from build123d import *

# Parameters (mm, degrees)
SKETCH1_R           = 4.5
BOSS_EXTRUDE2_DEPTH = 5
SKETCH2_W           = 5
SKETCH2_H           = 2.5
BOSS_EXTRUDE3_DEPTH = 10
SKETCH3_W           = 10
SKETCH3_H           = 2.5
BOSS_EXTRUDE4_DEPTH = 5
SKETCH4_W           = 10
SKETCH4_H           = 2.5
BOSS_EXTRUDE5_DEPTH = 5
SKETCH5_R           = 1.65
CUT_EXTRUDE1_DEPTH  = 5
CHAMFER1_SIZE       = 5.773502692
CHAMFER1_SIZE_2     = 10
FILLET1_R           = 2
FILLET2_R           = 5
FILLET3_R           = 2
FILLET4_R           = 2
FILLET5_R           = 10
FILLET6_R           = 3
SKETCH6_R           = 1.65
SKETCH6_W           = 36.073404507
SKETCH6_H           = 7.954648173
CUT_EXTRUDE2_DEPTH  = 5
FILLET10_R          = 2


with BuildPart() as part:
    # Sketch1 → Boss-Extrude2 (new body)
    with BuildSketch(Plane.XY):
        with BuildLine():
            Line((-7.5, 20), (-5.870329309, 16.740658618))
            ThreePointArc((-5.870329309, 16.740658618), (0, 21.5), (5.870329309, 16.740658618))
            Line((5.870329309, 16.740658618), (7.5, 20))
            Line((7.5, 20), (12.5, 20))
            Line((12.5, 20), (12.5, 15))
            Line((12.5, 15), (5, 0))
            Line((5, 0), (12.5, -15))
            Line((12.5, -15), (12.5, -20))
            Line((12.5, -20), (7.5, -20))
            Line((7.5, -20), (0, -5))
            Line((0, -5), (-7.5, -20))
            Line((-7.5, -20), (-12.5, -20))
            Line((-12.5, -20), (-12.5, -15))
            Line((-12.5, -15), (-5, 0))
            Line((-5, 0), (-12.5, 15))
            Line((-12.5, 15), (-12.5, 20))
            Line((-12.5, 20), (-7.5, 20))
        make_face()
        with Locations((0, 15.5)):
            Circle(SKETCH1_R, mode=Mode.SUBTRACT)
    extrude(amount=BOSS_EXTRUDE2_DEPTH)

    # Sketch2 → Boss-Extrude3 (add)
    with BuildSketch(Plane.XY.offset(5)):
        with Locations((-10, -18.75)):
            Rectangle(SKETCH2_W, SKETCH2_H)
        with Locations((10, -18.75)):
            Rectangle(SKETCH2_W, SKETCH2_H)
    extrude(amount=BOSS_EXTRUDE3_DEPTH)

    # Sketch3 → Boss-Extrude4 (add)
    with BuildSketch(Plane(origin=(12.5, 0, 0), x_dir=(0, 0, -1), z_dir=(1, 0, 0))):
        with Locations((-5, -18.75)):
            Rectangle(SKETCH3_W, SKETCH3_H)
    extrude(amount=BOSS_EXTRUDE4_DEPTH)

    # Sketch4 → Boss-Extrude5 (add)
    with BuildSketch(Plane.ZY.offset(12.5)):
        with Locations((5, -18.75)):
            Rectangle(SKETCH4_W, SKETCH4_H)
    extrude(amount=BOSS_EXTRUDE5_DEPTH)

    # Sketch5 → Cut-Extrude1 (cut)
    with BuildSketch(Plane(origin=(0, -17.5, 0), x_dir=(1, 0, 0), z_dir=(0, 1, 0))):
        with Locations(Location((-15, -3, 0), (0, 0, 270))):
            Circle(SKETCH5_R)
        with Locations(Location((-10, -12, 0), (0, 0, 270))):
            Circle(SKETCH5_R)
        with Locations(Location((10, -12, 0), (0, 0, 270))):
            Circle(SKETCH5_R)
        with Locations(Location((15, -3, 0), (0, 0, 270))):
            Circle(SKETCH5_R)
    extrude(amount=-CUT_EXTRUDE1_DEPTH, mode=Mode.SUBTRACT)

    # Chamfer1
    # the kernel refuses this chamfer: 10, 5.773502692 mm, written as the material it takes off along each edge
    with BuildSketch(Plane(origin=(17.5, -45.870857546, 10), x_dir=(0.05789386240267053, 0, -0.9983227437537926), z_dir=(0, 1, 0))) as chamfer1_piece_1_section:
        Polygon((CHAMFER1_SIZE * 0.998322743736, CHAMFER1_SIZE * 0.0578938624016), (-CHAMFER1_SIZE_2 * 0.0578938624027, CHAMFER1_SIZE_2 * 0.998322743754), (0, 0), align=None)
    chamfer1_piece_1 = extrude(amount=54.241715093, mode=Mode.PRIVATE)
    chamfer1_piece_1 = split(chamfer1_piece_1, bisect_by=Plane(origin=(12.5, -18.75, 7.760588383), z_dir=(1, 0, 0)), keep=Keep.TOP, mode=Mode.PRIVATE)
    add(chamfer1_piece_1, mode=Mode.SUBTRACT)
    with BuildSketch(Plane(origin=(-17.5, -45.870857546, 10), x_dir=(-0.05789386240267053, 0, -0.9983227437537926), z_dir=(0, 1, 0))) as chamfer1_piece_2_section:
        Polygon((CHAMFER1_SIZE * 0.998322743736, -CHAMFER1_SIZE * 0.0578938624016), (-CHAMFER1_SIZE_2 * 0.0578938624027, -CHAMFER1_SIZE_2 * 0.998322743754), (0, 0), align=None)
    chamfer1_piece_2 = extrude(amount=54.241715093, mode=Mode.PRIVATE)
    chamfer1_piece_2 = split(chamfer1_piece_2, bisect_by=Plane(origin=(-12.5, -18.75, 7.760588383), z_dir=(-1, 0, 0)), keep=Keep.TOP, mode=Mode.PRIVATE)
    add(chamfer1_piece_2, mode=Mode.SUBTRACT)

    # Fillet1
    fillet1_edges = [part.edges().sort_by_distance(p)[0] for p in [
        (12.5, -18.75, 15),
        (7.5, -18.75, 15),
        (-7.5, -18.75, 15),
        (-12.5, -18.75, 15),
    ]]
    fillet(fillet1_edges, radius=FILLET1_R)

    # Fillet2
    fillet2_edges = [part.edges().sort_by_distance(p)[0] for p in [
        (12.5, -18.75, 7.113248654),
        (-12.5, -18.75, 7.113248654),
    ]]
    fillet(fillet2_edges, radius=FILLET2_R)

    # Fillet3
    fillet3_edges = [part.edges().sort_by_distance(p)[0] for p in [
        (17.5, -18.75, 4.226497308),
        (-17.5, -18.75, 4.226497308),
    ]]
    fillet(fillet3_edges, radius=FILLET3_R)

    # Fillet4
    # the kernel refuses this fillet: 2 mm, written as the material it adds along each edge
    with BuildSketch(Plane(origin=(-5.870329309, 16.740658618, 0), x_dir=(-0.4472135954999439, 0.894427190999923, 0), z_dir=(0, 0, 1))) as fillet4_piece_1:
        with BuildLine():
            CenterArc((3.795112325, -1.99428722), FILLET4_R, 94.331614503, 105.404093699)
            Line((1.912591774, -2.669651103), (1.874941363, -2.683158381))
            ThreePointArc((1.874941363, -2.683158381), (1.109985705, -1.224719073), (-0.024899799, -0.031304952))
            Line((-0.024899799, -0.031304952), (0, 0.04))
            ThreePointArc((0, 0.04), (1.822027223, 0.04), (3.641033289, 0.039885744))
            Line((3.641033289, 0.039885744), (3.644054446, 0))
        make_face()
    extrude(amount=5)
    with BuildSketch(Plane(origin=(5.870329309, 16.740658618, 0), x_dir=(-0.46663943526551355, 0.8844476454008358, 0), z_dir=(0, 0, 1))) as fillet4_piece_2:
        with BuildLine():
            CenterArc((3.831402307, -1.923646391), FILLET4_R, 105.88286544, 105.404093699)
            Line((2.1222482, -2.962295628), (2.088065118, -2.983068612))
            ThreePointArc((2.088065118, -2.983068612), (1.02860762, -1.504443275), (-0.03251648, -0.023295461))
            Line((-0.03251648, -0.023295461), (0.010946864, 0.038472928))
            ThreePointArc((0.010946864, 0.038472928), (1.64202956, -0.189060828), (3.273112257, 0.038472928))
            Line((3.273112257, 0.038472928), (3.284059121, 0))
        make_face()
    extrude(amount=5)
    with BuildSketch(Plane(origin=(0, -5, 0), x_dir=(-0.4472135954999584, -0.8944271909999157, 0), z_dir=(0, 0, 1))) as fillet4_piece_3:
        with BuildLine():
            CenterArc((FILLET4_R * 2, FILLET4_R), FILLET4_R, 143.130102354, 126.869897646)
            Line((FILLET4_R * 1.2, FILLET4_R * 1.6), (FILLET4_R * 1.184, FILLET4_R * 1.612))
            Line((FILLET4_R * 1.184, FILLET4_R * 1.612), (-FILLET4_R * 0.016, FILLET4_R * 0.012))
            Line((-FILLET4_R * 0.016, FILLET4_R * 0.012), (0, -FILLET4_R * 0.02))
            Line((0, -FILLET4_R * 0.02), (FILLET4_R * 2, -FILLET4_R * 0.02))
            Line((FILLET4_R * 2, -FILLET4_R * 0.02), (FILLET4_R * 2, 0))
        make_face()
    extrude(amount=5)

    # Fillet5
    fillet5_edges = [part.edges().sort_by_distance(p)[0] for p in [
        (5, 0, 2.5),
        (-5, 0, 2.5),
    ]]
    fillet(fillet5_edges, radius=FILLET5_R)

    # Fillet6
    fillet6_edges = [part.edges().sort_by_distance(p)[0] for p in [
        (7.5, 20, 2.5),
        (12.5, 20, 2.5),
        (12.5, 15, 2.5),
        (-12.5, 15, 2.5),
        (-12.5, 20, 2.5),
        (-7.5, 20, 2.5),
    ]]
    fillet(fillet6_edges, radius=FILLET6_R)

    # Sketch6 → Cut-Extrude2 (cut)
    with BuildSketch(Plane(origin=(0, -17.5, 0), x_dir=(1, 0, 0), z_dir=(0, 1, 0))):
        with Locations(Location((-10, -7.5, 0), (0, 0, 270))):
            Circle(SKETCH6_R)
        with Locations(Location((10, -7.5, 0), (0, 0, 270))):
            Circle(SKETCH6_R)
        with Locations((1.341190681, -13.977324087)):
            Rectangle(SKETCH6_W, SKETCH6_H)
    extrude(amount=-CUT_EXTRUDE2_DEPTH, mode=Mode.SUBTRACT)

    # Fillet10
    fillet10_edges = [part.edges().sort_by_distance(p)[0] for p in [
        (12.5, -18.75, 10),
        (-12.5, -18.75, 10),
        (7.5, -18.75, 10),
        (-7.5, -18.75, 10),
    ]]
    fillet(fillet10_edges, radius=FILLET10_R)


solid = part.part
Model file for the job. Use its own axes, mm. A direction names the side the tool comes from. Coordinates: 2 decimals unless noted, no trailing zeros. Write each loop counter-clockwise with the first axis right and the second up, starting at its lowest first coordinate (ties: lowest second). Pieces come first, ordered by that corner, then holes. Notation, with made-up numbers: (14.25, 10.5) -> (26.25, 10.5) arc R25 cw to (26.25, 28.5) -> close; hole circle Ø7 at (-5.75, 55). An arc over 180 degrees is marked (long way). One line per item, written item: value. Start each with the question number.
1) Slice it at B-B on y = -6. Write the cut outline in (x, z), then the cut area to 3 significant figures.
2) Slice it at C-C on x = -10. Write the cut outline in (y, z), then the cut area to 3 significant figures.
3) Slice it at D-D on z = 2.25. Count the separate pieces of the cut face and the enclosed holes in it, then the cut area to 3 significant figures.
4) Pull direction Z, two halves, no side cores. Call faces 1 (the face through (-11, -18.73, 6.19)), 2 (the face through (13, -17.5, 5)), 3 (the face through (10, -19, 10)): +Z half, -Z half, draft (parallel to the pull), parting line (faces both ways), or undercut.
5) Probe probe 1 along X at (y, z) = (-18.55, 7.5); probe 2 along Z at (x, y) = (7.5, -7.5); probe 3 along Y at (x, z) = (-13, 3). List the from-to ranges inside material, lowest first.
6) Which spindle directions (+Z, -Z, +X, -X, +Y, -Y) get a long thin tool onto all of the face, cutting with end or side? Do faces 4 (the face through (-9.7, 9.4, 2.5)), 5 (the face through (12.5, 16, 2)), 6 (the face through (10, -10, 2)), 7 (the face through (-12.5, 16, 2)). Say none if no direction does.
7) Slice it at A-A on x = 0. Write the cut outline in (y, z).
8) Flat gauge pins, fed straight in: pin 1 Ø1 at (y, z) = (16, 4.5) entering from -X; pin 2 Ø1.2 at (y, z) = (-18.5, 6.5) entering from -X; pin 3 Ø4.5 at (x, z) = (15, 3) entering from +Y. Where does each tip first touch, or does it go through?
Answers follow:
1. outline: (-8, 0) -> (8, 0) -> (8, 5) -> (-8, 5) -> close
1. area: 80.0 mm2
2. outline: (-20, 0) -> (-10, 0) -> (-10, 5) -> (-17.5, 5) -> (-17.5, 5.85) -> (-20, 5.85) -> close; (-20, 9.15) -> (-17.5, 9.15) -> (-17.5, 10) -> (-20, 10) -> close; (10, 0) -> (19.96, 0) -> (19.96, 5) -> (10, 5) -> close
2. area: 104 mm2
3. separate pieces: 3
3. enclosed holes: 1
3. area: 619 mm2
4. face 1: undercut
4. face 2: draft
4. face 3: +Z half
5. probe 1: -13.17 to -11.65, -8.35 to -7.5, 7.5 to 8.35, 11.65 to 13.17
5. probe 2: 0 to 5
5. probe 3: -20 to -17.5
6. face 4: +Z, -Z, -X
6. face 5: +Z, -Z, +X, +Y
6. face 6: +Z, -Z, +X
6. face 7: +Z, -Z, -X, +Y
7. outline: (-7.47, 0) -> (11, 0) -> (11, 5) -> (-7.47, 5) -> close; (20, 0) -> (21.5, 0) -> (21.5, 5) -> (20, 5) -> close
8. pin 1: x = -12.5
8. pin 2: x = -14.64
8. pin 3: y = -17.5
